from build123d import *

# Parameters (mm, degrees)
SM_BASE_FLANGE_1_DEPTH = 367.5
CUT_EXTRUDE_1337_DEPTH = 40.5
CUT_EXTRUDE_2_DEPTH    = 41
CUT_EXTRUDE_START      = -41
CUT_EXTRUDE_3_DEPTH    = 41
SKETCH_6_W             = 40
SKETCH_6_H             = 6
EXTRUDE_4_DEPTH        = 12
EXTRUDE_START          = 42.5
EXTRUDE_5_DEPTH        = 42.5
EXTRUDE_6_DEPTH        = 42.5
CHAMFER_1_SIZE         = 10
M6X1_01_D              = 5
M6X1_01_CSINK_D        = 6.5
M6X1_01_CSINK_ANGLE    = 90
SKETCH_10_R            = 41
CUT_EXTRUDE_7_DEPTH    = 376.015749694
M5X0_81_D              = 4.2
M5X0_81_DEPTH          = 4.5
M5X0_81_CSINK_D        = 5.5
M5X0_81_CSINK_ANGLE    = 90
M6X1_02_D              = 5
M6X1_02_DEPTH          = 6
M6X1_02_CSINK_D        = 6.5
M6X1_02_CSINK_ANGLE    = 90
CUT_EXTRUDE_8_REACH    = 386.75
SKETCH_17_R            = 3.25


# Sheet-metal steps are written as plain solids
with BuildPart() as part:
    # Sketch 1 → Базовая кромка1 (new, symmetric)
    with BuildSketch(Plane(origin=(0, 0, 0), x_dir=(0, 0, -1), z_dir=(1, 0, 0))):
        with BuildLine():
            Line((23, 53.25), (-11, 53.25))
            ThreePointArc((-11, 53.25), (-19.485281374, 49.735281374), (-23, 41.25))
            Line((-23, 41.25), (-23, -41.25))
            ThreePointArc((-23, -41.25), (-19.485281374, -49.735281374), (-11, -53.25))
            Line((-11, -53.25), (23, -53.25))
            Line((23, -53.25), (23, -47.25))
            Line((23, -47.25), (-11, -47.25))
            ThreePointArc((-11, -47.25), (-15.242640687, -45.492640687), (-17, -41.25))
            Line((-17, -41.25), (-17, 41.25))
            ThreePointArc((-17, 41.25), (-15.242640687, 45.492640687), (-11, 47.25))
            Line((-11, 47.25), (23, 47.25))
            Line((23, 47.25), (23, 53.25))
        make_face()
    extrude(amount=SM_BASE_FLANGE_1_DEPTH, both=True)

    # Эскиз3 → Cut-Extrude 1337 (cut)
    with BuildSketch(Plane(origin=(0, 0, -23), x_dir=(-1, 0, 0), z_dir=(0, 0, -1))):
        with BuildLine():
            Line((-45, -41.25), (45, -41.25))
            ThreePointArc((45, -41.25), (47.121320344, -40.371320344), (48, -38.25))
            Line((48, -38.25), (48, 45.75))
            ThreePointArc((48, 45.75), (47.121320344, 47.871320344), (45, 48.75))
            Line((45, 48.75), (-45, 48.75))
            ThreePointArc((-45, 48.75), (-47.121320344, 47.871320344), (-48, 45.75))
            Line((-48, 45.75), (-48, -38.25))
            ThreePointArc((-48, -38.25), (-47.121320344, -40.371320344), (-45, -41.25))
        make_face()
    extrude(amount=-CUT_EXTRUDE_1337_DEPTH, mode=Mode.SUBTRACT)

    # Эскиз4 → Вытянуть2 (cut)
    with BuildSketch(Plane(origin=(367.5, 0, 0), x_dir=(0, 0, -1), z_dir=(1, 0, 0))):
        with BuildLine():
            Line((-11, 47.25), (-11, 53.25))
            ThreePointArc((-11, 53.25), (-19.485281374, 49.735281374), (-23, 41.25))
            Line((-23, 41.25), (-23, -41.25))
            ThreePointArc((-23, -41.25), (-19.485281374, -49.735281374), (-11, -53.25))
            Line((-11, -53.25), (23, -53.25))
            Line((23, -53.25), (23, -47.25))
            Line((23, -47.25), (-11, -47.25))
            ThreePointArc((-11, -47.25), (-15.242640687, -45.492640687), (-17, -41.25))
            Line((-17, -41.25), (-17, 41.25))
            ThreePointArc((-17, 41.25), (-15.242640687, 45.492640687), (-11, 47.25))
        make_face()
    extrude(amount=-CUT_EXTRUDE_2_DEPTH, mode=Mode.SUBTRACT)

    # Эскиз5 → Вытянуть3 (cut)
    with BuildSketch(Plane.ZY.offset(367.5).offset(CUT_EXTRUDE_START)):
        with BuildLine():
            Line((11, 53.25), (11, 47.25))
            ThreePointArc((11, 47.25), (15.242640687, 45.492640687), (17, 41.25))
            Line((17, 41.25), (17, -41.25))
            ThreePointArc((17, -41.25), (15.242640687, -45.492640687), (11, -47.25))
            Line((11, -47.25), (-23, -47.25))
            Line((-23, -47.25), (-23, -53.25))
            Line((-23, -53.25), (11, -53.25))
            ThreePointArc((11, -53.25), (19.485281374, -49.735281374), (23, -41.25))
            Line((23, -41.25), (23, 41.25))
            ThreePointArc((23, 41.25), (19.485281374, 49.735281374), (11, 53.25))
        make_face()
    extrude(amount=CUT_EXTRUDE_3_DEPTH, mode=Mode.SUBTRACT)

    # Эскиз6 → Вытянуть4 (add)
    with BuildSketch(Plane.XY.offset(11)):
        with Locations((-347.5, 50.25)):
            Rectangle(SKETCH_6_W, SKETCH_6_H)
        with Locations((347.5, 50.25)):
            Rectangle(SKETCH_6_W, SKETCH_6_H)
    extrude(amount=EXTRUDE_4_DEPTH)

    # Эскиз8 → Вытянуть5 (add)
    with BuildSketch(Plane(origin=(326.5, 0, 0), x_dir=(0, 0, -1), z_dir=(1, 0, 0)).offset(EXTRUDE_START)):
        with BuildLine():
            Line((-17, -41.25), (-17, 38.75))
            Line((-17, 38.75), (-23, 38.75))
            Line((-23, 38.75), (-23, -41.25))
            ThreePointArc((-23, -41.25), (-22.916902714, -42.659762285), (-22.668761717, -44.05))
            Line((-22.668761717, -44.05), (-16.306599665, -44.05))
            ThreePointArc((-16.306599665, -44.05), (-16.824070655, -42.692290195), (-17, -41.25))
        make_face()
    extrude(amount=-EXTRUDE_5_DEPTH)

    # Эскиз9 → Вытянуть6 (add)
    with BuildSketch(Plane.ZY.offset(326.5)):
        with BuildLine():
            Line((17, 38.75), (17, -41.25))
            ThreePointArc((17, -41.25), (16.824070655, -42.692290195), (16.306599665, -44.05))
            Line((16.306599665, -44.05), (22.668761717, -44.05))
            ThreePointArc((22.668761717, -44.05), (22.916902714, -42.659762285), (23, -41.25))
            Line((23, -41.25), (23, 38.75))
            Line((23, 38.75), (17, 38.75))
        make_face()
    extrude(amount=EXTRUDE_6_DEPTH)

    # Фаска1
    chamfer_1_edges = [part.edges().sort_by_distance(p)[0] for p in [
        (-369, 38.75, 20),
        (-369, -44.05, 19.487680691),
        (369, 38.75, 20),
        (369, -44.05, 19.487680691),
    ]]
    chamfer(chamfer_1_edges, length=CHAMFER_1_SIZE)

    # Отверстие обработанное метчиком M6x1.01 (through all)
    with Locations(Plane(origin=(0, 0, 17.5), x_dir=(-1, 0, 0), z_dir=(0, 0, -1))):
        with Locations((-35.355339059, 39.105339059), (35.355339059, 39.105339059), (35.355339059, -31.605339059), (-35.355339059, -31.605339059)):
            CounterSinkHole(M6X1_01_D / 2, M6X1_01_CSINK_D / 2, counter_sink_angle=M6X1_01_CSINK_ANGLE)

    # Эскиз10 → Вытянуть7 (cut, through all)
    with BuildSketch(Plane(origin=(0, 0, 17.5), x_dir=(-1, 0, 0), z_dir=(0, 0, -1))):
        with Locations((0, 3.75)):
            Circle(SKETCH_10_R)
    extrude(amount=-CUT_EXTRUDE_7_DEPTH, mode=Mode.SUBTRACT)

    # Отверстие обработанное метчиком M5x0.81
    with Locations(Plane(origin=(0, 53.25, 0), x_dir=(-1, 0, 0), z_dir=(0, 1, 0))):
        with Locations((42, -9), (-42, -9), (-14, -9), (14, -9)):
            CounterSinkHole(M5X0_81_D / 2, M5X0_81_CSINK_D / 2, depth=M5X0_81_DEPTH, counter_sink_angle=M5X0_81_CSINK_ANGLE)

    # Отверстие обработанное метчиком M6x1.02
    with Locations(Plane.XZ.offset(53.25)):
        with Locations((0, -17), (-42, -17), (42, -17)):
            CounterSinkHole(M6X1_02_D / 2, M6X1_02_CSINK_D / 2, depth=M6X1_02_DEPTH, counter_sink_angle=M6X1_02_CSINK_ANGLE)

    # Эскиз17 → Вытянуть8 (cut, up to next)
    with BuildSketch(Plane(origin=(0, 53.25, 0), x_dir=(1, 0, 0), z_dir=(0, 1, 0)), mode=Mode.PRIVATE) as cut_extrude_8_sk1:
        with Locations(Location((-112.5, 7.5, 0), (0, 0, 270))):
            Circle(SKETCH_17_R)
    cut_extrude_8_tool1 = extrude(cut_extrude_8_sk1.sketch, amount=-CUT_EXTRUDE_8_REACH, mode=Mode.PRIVATE) & part.part
    # Эскиз17 → Вытянуть8 (cut, up to next)
    with BuildSketch(Plane(origin=(0, 53.25, 0), x_dir=(1, 0, 0), z_dir=(0, 1, 0)), mode=Mode.PRIVATE) as cut_extrude_8_sk2:
        with Locations(Location((112.5, 7.5, 0), (0, 0, 270))):
            Circle(SKETCH_17_R)
    cut_extrude_8_tool2 = extrude(cut_extrude_8_sk2.sketch, amount=-CUT_EXTRUDE_8_REACH, mode=Mode.PRIVATE) & part.part
    add(cut_extrude_8_tool1.solids().sort_by_distance((-112.5, 53.25, -7.5))[0], mode=Mode.SUBTRACT)
    add(cut_extrude_8_tool2.solids().sort_by_distance((112.5, 53.25, -7.5))[0], mode=Mode.SUBTRACT)


solid = part.part
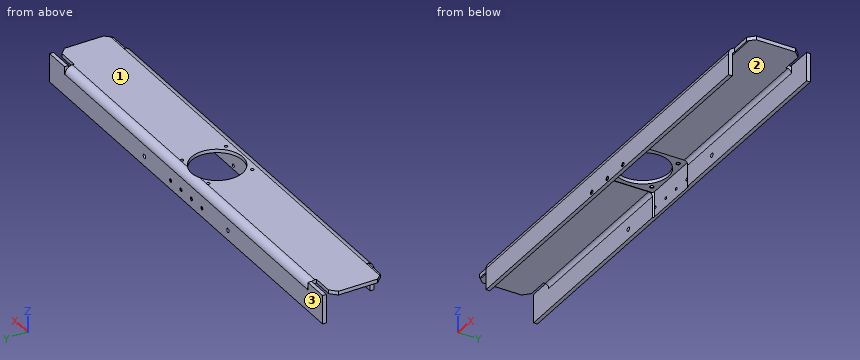
Read the model definition and answer for the solid it produces. Units are mm, in the model's axes. Face numbers are marked on the shaded views. Round coordinates to 2 decimals unless told otherwise and drop trailing zeros. Loops run counter-clockwise (first coordinate to the right, second up) from the corner with the lowest first, then second, coordinate; pieces in that order, holes last.
Q1. Section A-A on y = -4.5 is taken. Write down the section's boundary in (x, z).
Q2. Determine the mould class of the marked faces 1, 2 and 3 for opening direction Y: released by +Y, released by -Y, zero draft, split by the parting line, or undercut.
Q3. Each of these flat-tipped pins is pushed along its axis until it touches: pin 1 (5 mm diameter, centred on x = 289.5, y = -9.5, fed in from -Z); pin 2 (4 mm diameter, centred on x = 42, z = -17, fed in from -Y); pin 3 (6 mm diameter, centred on x = -35.36, y = -31.61, fed in from -Z). Where does it stop, or does it pass through?
Q4. Section B-B on x = 102 is taken. Write down the section's boundary in (y, z).
Q5. Consider probe 1 along Y at (x, z) = (-273.5, -6); probe 2 along Z at (x, y) = (48.5, 28.5). Determine where each line is inside the solid, lowest interval first.
Output:
1. outline: (-369, 17) - (-48, 17) - (-48, 17.5) - (-40.16, 17.5) - (-40.16, 23) - (-369, 23) - close; (40.16, 17.5) - (48, 17.5) - (48, 17) - (369, 17) - (369, 23) - (40.16, 23) - close
2. face 1: zero draft
2. face 2: undercut
2. face 3: released by +Y
3. pin 1: stops at z = 17
3. pin 2: stops at y = 48.75
3. pin 3: stops at z = 17.74
4. outline: (-53.25, -23) - (-47.25, -23) - (-47.25, 11) arc R6 cw to (-41.25, 17) - (41.25, 17) arc R6 cw to (47.25, 11) - (47.25, -23) - (53.25, -23) - (53.25, 11) arc R12 ccw to (41.25, 23) - (-41.25, 23) arc R12 ccw to (-53.25, 11) - close
5. probe 1: y = -53.25 to -47.25, 47.25 to 53.25
5. probe 2: z = 17 to 23
